Source: three-view drawing plus pictorial views. Frame: mm from the lowest corner of the part. A direction names the side the tool comes from. Give positions to 0.01 mm unless a question says otherwise; leave off trailing zeros. Loops run counter-clockwise (first coordinate to the right, second up) from the corner with the lowest first, then second, coordinate; pieces in that order, holes last. Notation, with made-up numbers: (81, 34.5) - (90, 34.5) arc R27 cw to (90, 66.5) - close; hole circle Ø10 at (47.5, -23.5). An arc over 180 degrees is marked (long way). Answer as a JSON object with one key per item and string values. Group by question number.
(1) Access query for the marked faces 5 and 6. Directions: +Z, -Z, +X, -X, +Y, -Y. A direction counts if a zero-diameter tool reaches every point of the face in a straight line with its end or side. Return the directions, or none.
(2) Mould query, pull axis X, two halves, no side actions, for the marked faces 1, 2, 3 and 4. Classes: +X half, -X half, draft (parallel to the pull), parting line (faces both ways), or undercut.
(3) Section query A-A (z = 8.5). Return loops of the section in (x, y).
(4) Material intervals for L1, parallel to X at y = 57, z = 48.5, sorted ascending.
(5) Pin query (flat end, axial travel): P1, Ø19, axis at y = 82.5, z = 47.5, coming from the +X side; P2, Ø19, axis at y = 397.5, z = 26.5, coming from the -X side. Return the tip coordinate at first contact, or that it passes through.
(6) Section query B-B (y = 97). Return loops of the section in (x, z), plus the area to 3 significant figures.
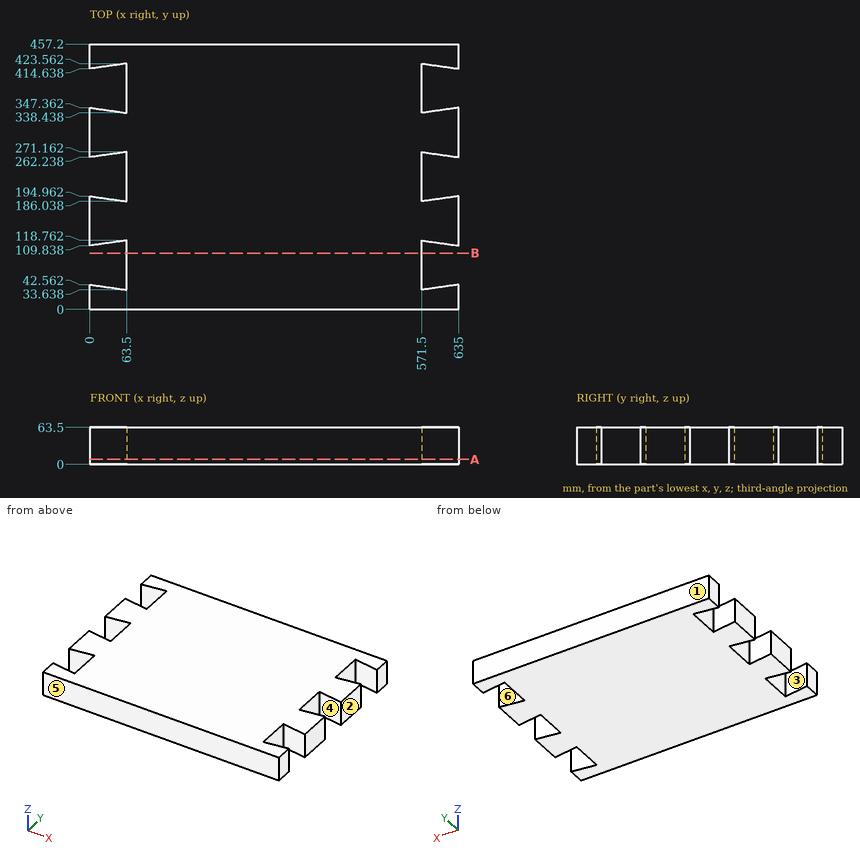
Recorded:
{
 "1": {"face 5": "+Z, -Z, +X, -X, -Y", "face 6": "+Z, -Z"},
 "2": {"face 1": "draft", "face 2": "+X half", "face 3": "undercut", "face 4": "undercut"},
 "3": {"outline": "(0, 0) - (635, 0) - (635, 42.56) - (571.5, 33.64) - (571.5, 118.76) - (635, 109.84) - (635, 194.96) - (571.5, 186.04) - (571.5, 271.16) - (635, 262.24) - (635, 347.36) - (571.5, 338.44) - (571.5, 423.56) - (635, 414.64) - (635, 457.2) - (0, 457.2) - (0, 414.64) - (63.5, 423.56) - (63.5, 338.44) - (0, 347.36) - (0, 262.24) - (63.5, 271.16) - (63.5, 186.04) - (0, 194.96) - (0, 109.84) - (63.5, 118.76) - (63.5, 33.64) - (0, 42.56) - close"},
 "4": {"L1": "x = 63.5 to 571.5"},
 "5": {"P1": "stops at x = 571.5", "P2": "stops at x = 63.5"},
 "6": {"outline": "(63.5, 0) - (571.5, 0) - (571.5, 63.5) - (63.5, 63.5) - close", "area": "32,300 mm^2"}
}
